from build123d import *

# Parameters (mm, degrees)
F0_R     = 7
F1_DEPTH = 10
F2_R     = 3.625
F3_DEPTH = 4
F4_R     = 2.1
F5_DEPTH = 10.001


with BuildPart() as f1:
    # F0 (on Right) → F1 (new body)
    with BuildSketch(Plane.YZ):
        Circle(F0_R)
    extrude(amount=F1_DEPTH)

    # F2 (on face) → F3 (cut)
    with BuildSketch(Plane(origin=(0, 0, 0), x_dir=(0, -1, 0), z_dir=(-1, 0, 0))):
        Circle(F2_R)
    extrude(amount=-F3_DEPTH, mode=Mode.SUBTRACT)

    # F4 (on face) → F5 (cut, through all)
    with BuildSketch(Plane.YZ.offset(10)):
        Circle(F4_R)
    extrude(amount=-F5_DEPTH, mode=Mode.SUBTRACT)


solid = f1.part
Could you check a few things on this model? Use its own coordinates, in mm. A direction names the side the tool comes from. Coordinates: 2 decimals unless noted, no trailing zeros. Order: outer loops, then holes, each group sorted by start corner. A loop starts at its lowest first (then second) coordinate and runs counter-clockwise, first axis right, second up.
Q1. Will these pins go through, and if not, where does the flat tip stop? pin 1 (4 mm diameter, centred on x = 3, y = -2.5, fed in from +Z); pin 2 (1 mm diameter, centred on x = 6.5, z = 5, fed in from +Y); pin 3 (1 mm diameter, centred on x = 6, y = 1.5, fed in from +Z).
Q2. Suppose I cut it at D-D on z = 2.75. Please give me the cut outline in (x, y), and give its area (3 significant figures).
Q3. Thinking about a two-plate mould opening in Z: for faces 3 (the flat face through (0, 3, -3)), 4 (the cylindrical face through (4.93, 6.466, -2.681)), 5 (the cylindrical face through (7.042, 2.003, 0.631)), which applies, released by +Z, released by -Z, zero draft, split by the parting line, or undercut?
Q4. Please list where these lines run through material, in increasing order: L1, parallel to Z at x = 7.95, y = 0; L2, parallel to Z at x = 4.5, y = 1; L3, parallel to Y at x = 2.5, z = -0.25.
Q5. Which directions (+Z, -Z, +X, -X, +Y, -Y) give clear straight access to the entire face, cutting with the end or side of a thin tool? Please do faces 1 (the flat face through (4, -2, -2)), 2 (the flat face through (10, 1.5, 1.7)).
Q6. Suppose I cut it at A-A on y = 0. Please give me the cut outline in (x, z) (3 decimals).
Q7. Suppose I cut it at C-C on x = 2.75. Please give me the cut outline in (y, z) (3 decimals), and give its area (3 significant figures).
Answer:
1. pin 1: stops at z = 6.98
1. pin 2: stops at y = 5.36
1. pin 3: stops at z = 6.93
2. outline: (0, -6.44) - (10, -6.44) - (10, 6.44) - (0, 6.44) - (0, 2.36) - (4, 2.36) - (4, -2.36) - (0, -2.36) - close
2. area: 110 mm2
3. face 3: zero draft
3. face 4: split by the parting line
3. face 5: undercut
4. L1: z = -7 to -2.1, 2.1 to 7
4. L2: z = -6.93 to -1.85, 1.85 to 6.93
4. L3: y = -7 to -3.62, 3.62 to 7
5. face 1: -X
5. face 2: +Z, -Z, +X, +Y, -Y
6. outline: (0, -7) - (10, -7) - (10, -2.1) - (4, -2.1) - (4, -3.625) - (0, -3.625) - close; (0, 3.625) - (4, 3.625) - (4, 2.1) - (10, 2.1) - (10, 7) - (0, 7) - close
7. outline: circle Ø14 at (0, 0); hole circle Ø7.25 at (0, 0)
7. area: 113 mm2
